Source: CAD feature listing. Evaluate the final solid. Frame: model axes, mm. A direction names the side the tool comes from. Round coordinates to 2 decimals unless told otherwise and drop trailing zeros. Order: outer loops, then holes, each group sorted by start corner. A loop starts at its lowest first (then second) coordinate and runs counter-clockwise, first axis right, second up. Notation, with made-up numbers: M 13,75.25 L 46,75.25 A25 ccw 46,114.25 Z; hole C 33,3.25 d4. An arc over 180 degrees is marked long. Answer as CSV lines item,"result". Start each with the question number.
Item 1: Set-up query: faces 1 (the face through (11, 39, 1)), 2 (the face through (17.9, 39.1, 0.5)), 3 (the face through (11.6, 37.6, 1.2)). Return all of +Z, -Z, +X, -X, +Y, -Y with unobstructed straight access to the full face (end or side cutting, diameter ignored); none if empty.
Item 2: First-contact query: P1, Ø0.9, axis at x = 13, y = 39.5, coming from the +Z side; P2, Ø2, axis at x = 17.5, y = 35, coming from the -Z side. Flat tips, straight axial feed; report the tip coordinate or a pass-through.
Item 3: Section query B-B on z = 0.35. Return the cut outline in (x, y), plus the area to 3 significant figures.
Item 4: Line query: line 1 (Z direction, x = 9, y = 38); line 2 (Y direction, x = 2.25, z = 1.6); line 3 (X direction, y = 7, z = 0.9). Output: solid intervals per line, ascending. Write a range as [from, to].
Autodesk Inventor part; units mm, degrees
ref_plane "YZ Plane" through (0, 0, 0) normal (1, 0, 0) x (0, 1, 0)
ref_plane "XZ Plane" through (0, 0, 0) normal (0, 1, 0) x (-1, 0, 0)
ref_plane "XY Plane" through (0, 0, 0) normal (0, 0, 1) x (1, 0, 0)
sketch "Skizze1" plane through (0, 0, 0) normal (0, 0, 1) x (1, 0, 0)
  line L0 (3.4, 37.6) -> (-3, 37.6)
  line L1 (-3, 37.6) -> (-3, 3)
  arc A0 (-3, 3) -> (0, 0) centre (0, 3) ccw
  line L2 (0, 0) -> (22.8, 0)
  arc A1 (22.8, 0) -> (25.8, 3) centre (22.8, 3) ccw
  line L3 (25.8, 3) -> (25.8, 37.6)
  line L4 (25.8, 37.6) -> (19.4, 37.6)
  line L5 (19.4, 37.6) -> (16.4, 40.6)
  line L6 (16.4, 40.6) -> (6.4, 40.6)
  line L7 (6.4, 40.6) -> (3.4, 37.6)
  line L8 (-1.8, 35.6) -> (24.6, 35.6)
  line L9 (24.6, 35.6) -> (24.6, 9.2)
  line L10 (24.6, 9.2) -> (-1.8, 9.2)
  line L11 (-1.8, 9.2) -> (-1.8, 35.6)
  line L12 (24.6, 35.6) -> (-1.8, 35.6)
  line L13 (-1.8, 35.6) -> (-1.8, 9.2)
  line L14 (-1.8, 9.2) -> (24.6, 9.2)
  line L15 (24.6, 9.2) -> (24.6, 35.6)
  line L16 (24.6, 35.6) -> (-1.8, 35.6)
  line L17 (-3, 37.6) -> (3.4, 37.6)
  line L18 (-3, 3) -> (-3, 37.6)
  arc A2 (-3, 3) -> (0, 0) centre (0, 3) ccw
  line L19 (22.8, 0) -> (0, 0)
  arc A3 (22.8, 0) -> (25.8, 3) centre (22.8, 3) ccw
  line L20 (25.8, 37.6) -> (25.8, 3)
  line L21 (19.4, 37.6) -> (25.8, 37.6)
  line L22 (19.4, 37.6) -> (16.4, 40.6)
  line L23 (16.4, 40.6) -> (6.4, 40.6)
  line L24 (6.4, 40.6) -> (3.4, 37.6)
  circle A4 centre (4.1926, 4.6) radius 2
  line L25 (11.4, 35.6) -> (11.4, 0)
  circle A5 centre (18.6074, 4.6) radius 2
  point P0 (-3, 37.6)
  point P1 (-3, 3)
  point P2 (0, 0)
extrude "Extrusion1" add sketch "Skizze1" along normal blind 2 contours L7 L6 L5 L4 L3 A1 L2 A0 L1 L0 | L8 L25 L10 L11 | L8 L9 L10 L25 | A4 | A5
chamfer "Fase1" distance 2 angle 45 5 edges at (25.8, 20.3, 2) (24.9213, 0.8787, 2) (11.4, 0, 2) (-2.1213, 0.8787, 2) (-3, 20.3, 2)
sketch "Skizze2" plane through (0, 0, 2) normal (0, 0, 1) x (1, 0, 0)
  line L0 (-1, 3) -> (-1, 37.6)
  arc A0 (-1, 3) -> (0, 2) centre (0, 3) ccw
  line L1 (22.8, 2) -> (0, 2)
  arc A1 (22.8, 2) -> (23.8, 3) centre (22.8, 3) ccw
  line L2 (23.8, 37.6) -> (23.8, 3)
  line L3 (23.8, 37.6) -> (19.4, 37.6)
  line L4 (19.4, 37.6) -> (16.4, 40.6)
  line L5 (16.4, 40.6) -> (6.4, 40.6)
  line L6 (6.4, 40.6) -> (3.4, 37.6)
  line L7 (3.4, 37.6) -> (-1, 37.6)
  line L8 (6.4, 40.6) -> (3.4, 37.6)
  line L9 (3.4, 37.6) -> (19.4, 37.6)
  point P0 (0, 0)
extrude "Extrusion2" cut sketch "Skizze2" against normal blind 1 contours L6 L5 L4 L9
properties part number "gps-deckel"
Results:
1,face 1,"+Z, +X, -X, +Y"
1,face 2,"+Z, -Z, +X, +Y"
1,face 3,"+Z, +Y"
2,P1,"z = 1"
2,P2,"z = 0"
3,outline,"M -2.65,3 A2.65 ccw 0,0.35 L 22.8,0.35 A2.65 ccw 25.45,3 L 25.45,37.6 L 19.4,37.6 L 16.4,40.6 L 6.4,40.6 L 3.4,37.6 L -2.65,37.6 Z"
3,area,"1,080 mm^2"
4,line 1,"[0, 1]"
4,line 2,"[1.6, 37.6]"
4,line 3,"[-2.1, 24.9]"
